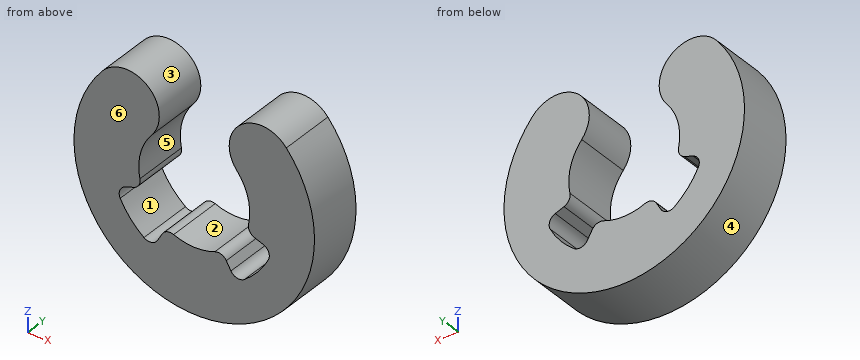
```python
from build123d import *

# Parameters (mm, degrees)
RESSALTO_EXTRUS_O1_DEPTH = 3


with BuildPart() as part:
    # Esboço1 → Ressalto-extrusão1 (new body)
    with BuildSketch(Plane(origin=(0, 0, 0), x_dir=(1, 0, 0), z_dir=(0, 1, 0))):
        with BuildLine():
            Line((-3.729289475, 1.357350364), (-3.255190725, 1.184792531))
            ThreePointArc((-3.255190725, 1.184792531), (-2.989342722, 0.958164276), (-2.93674354, 0.612811046))
            ThreePointArc((-2.93674354, 0.612811046), (-2.909531771, -0.731180466), (-2.298133329, -1.928362829))
            ThreePointArc((-2.298133329, -1.928362829), (-2.513832788, -4.393818921), (-4.97928888, -4.178119463))
            ThreePointArc((-4.97928888, -4.178119463), (0, 6.5), (4.97928888, -4.178119463))
            ThreePointArc((4.97928888, -4.178119463), (2.513832788, -4.393818921), (2.298133329, -1.928362829))
            ThreePointArc((2.298133329, -1.928362829), (2.909531771, -0.731180466), (2.93674354, 0.612811046))
            ThreePointArc((2.93674354, 0.612811046), (2.989342722, 0.958164276), (3.255190725, 1.184792531))
            Line((3.255190725, 1.184792531), (3.729289475, 1.357350364))
            ThreePointArc((3.729289475, 1.357350364), (4.023776667, 1.644680105), (4.003064329, 2.055596259))
            ThreePointArc((4.003064329, 2.055596259), (3.447199994, 2.892544244), (2.719491958, 3.585298243))
            ThreePointArc((2.719491958, 3.585298243), (2.318415204, 3.677050755), (1.984313483, 3.436931771))
            Line((1.984313483, 3.436931771), (1.732050808, 3))
            ThreePointArc((1.732050808, 3), (1.462701523, 2.777544409), (1.113461233, 2.785714286))
            ThreePointArc((1.113461233, 2.785714286), (0, 3), (-1.113461233, 2.785714286))
            ThreePointArc((-1.113461233, 2.785714286), (-1.462701523, 2.777544409), (-1.732050808, 3))
            Line((-1.732050808, 3), (-1.984313483, 3.436931771))
            ThreePointArc((-1.984313483, 3.436931771), (-2.318415204, 3.677050755), (-2.719491958, 3.585298243))
            ThreePointArc((-2.719491958, 3.585298243), (-3.447199994, 2.892544244), (-4.003064329, 2.055596259))
            ThreePointArc((-4.003064329, 2.055596259), (-4.023776667, 1.644680105), (-3.729289475, 1.357350364))
        make_face()
    extrude(amount=RESSALTO_EXTRUS_O1_DEPTH)


solid = part.part
```
Design review of the part built by this model. Coordinates are the model's own, in mm. Face numbers are marked on the shaded views. A direction names the side the tool comes from. Coordinates: 2 decimals unless noted, no trailing zeros. Write each loop counter-clockwise with the first axis right and the second up, starting at its lowest first coordinate (ties: lowest second). Pieces come first, ordered by that corner, then holes.
1) Add section C-C (x = 0). Write out the cut boundary in (y, z), plus the area to 3 significant figures.
2) Insertion check: pin 1 (1 mm diameter, centred on y = 2, z = -2, fed in from -X); pin 2 (4 mm diameter, centred on x = 0, z = 2.5, fed in from -Y). Each pin has a flat end and moves straight along its axis. Give the tip position at first contact, or say it passes through.
3) To check wall thickness, follow L1, parallel to X at y = 0.4, z = -3.5; L2, parallel to X at y = 1.45, z = -3.25; L3, parallel to X at y = 2.6, z = -2.25. State the ranges of each line that lie inside material, in increasing order.
4) Add section B-B (y = 0.2). Write out the cut boundary in (x, z).
5) Add section A-A (z = 0). Write out the cut boundary in (x, y).
6) Mouldability with a two-part tool opening along Z and no side actions: class the marked faces 3, 4, 5 and 6 as +Z half, -Z half, draft (parallel to the pull), parting line (faces both ways), or undercut.
7) Add section D-D (z = -2.25). Write out the cut boundary in (x, y), plus the area to 3 significant figures.
8) Machinability: for the marked faces 1 and 2, which of the approach directions +Z, -Z, +X, -X, +Y, -Y give a long, thin tool a straight path to every point of the face, cutting with its end or side? Answer none if there is none.
Check result:
1. outline: (0, -6.5) - (3, -6.5) - (3, -3) - (0, -3) - close
1. area: 10.5 mm2
2. pin 1: stops at x = -6.32
2. pin 2: stops at y = 0
3. L1: x = -5.48 to -2.83, -2.03 to 2.03, 2.83 to 5.48
3. L2: x = -5.63 to -3.11, -1.88 to 1.88, 3.11 to 5.63
3. L3: x = -6.1 to -3.9, 3.9 to 6.1
4. outline: (-4.98, 4.18) arc R6.5 ccw (long way) to (4.98, 4.18) arc R1.75 ccw to (2.3, 1.93) arc R3 cw to (2.94, -0.61) arc R0.5 ccw to (3.26, -1.18) - (3.73, -1.36) arc R0.5 cw to (4, -2.06) arc R4.5 cw to (2.72, -3.59) arc R0.5 cw to (1.98, -3.44) - (1.73, -3) arc R0.5 ccw to (1.11, -2.79) arc R3 cw to (-1.11, -2.79) arc R0.5 ccw to (-1.73, -3) - (-1.98, -3.44) arc R0.5 cw to (-2.72, -3.59) arc R4.5 cw to (-4, -2.06) arc R0.5 cw to (-3.73, -1.36) - (-3.26, -1.18) arc R0.5 ccw to (-2.94, -0.61) arc R3 cw to (-2.3, 1.93) arc R1.75 ccw to start
5. outline: (-6.5, 0) - (-3, 0) - (-3, 3) - (-6.5, 3) - close; (3, 0) - (6.5, 0) - (6.5, 3) - (3, 3) - close
6. face 3: undercut
6. face 4: parting line
6. face 5: undercut
6. face 6: draft
7. outline: (-6.1, 0) - (-3.9, 0) - (-3.9, 3) - (-6.1, 3) - close; (3.9, 0) - (6.1, 0) - (6.1, 3) - (3.9, 3) - close
7. area: 13.2 mm2
8. face 1: +Y, -Y
8. face 2: +Z, +Y, -Y
